Geometry: final body of the model. Coordinates: model frame, mm. Face numbers are marked on the shaded views. A direction names the side the tool comes from. Give positions to 0.01 mm unless a question says otherwise; leave off trailing zeros. Write each loop counter-clockwise with the first axis right and the second up, starting at its lowest first coordinate (ties: lowest second). Pieces come first, ordered by that corner, then holes. Notation, with made-up numbers: (12.25, -36.75) -> (42.25, -36.75) arc R27 ccw to (42.25, -12.75) -> close; hole circle Ø9 at (69, 80). An arc over 180 degrees is marked (long way). Answer in a Markdown table with one row per item. Add a question column.
Autodesk Inventor part; units mm, degrees
ref_plane "YZ Plane" through (0, 0, 0) normal (1, 0, 0) x (0, 1, 0)
ref_plane "XZ Plane" through (0, 0, 0) normal (0, 1, 0) x (-1, 0, 0)
ref_plane "XY Plane" through (0, 0, 0) normal (0, 0, 1) x (1, 0, 0)
sketch "Sketch1" plane through (0, 0, 0) normal (0, 1, 0) x (-1, 0, 0)
  circle A0 centre (0, 0) radius 9.25
  circle A1 centre (0, 0) radius 13.25
  dimension "d0" = 18.5
  dimension "d1" = 4
extrude "Extrusion1" add sketch "Sketch1" along normal blind 20
sketch "Sketch4" plane through (0, 0, 0) normal (0, -1, 0) x (1, 0, 0)
  circle A0 centre (0, 0) radius 13.25
  circle A1 centre (0, 0) radius 13.25
extrude "Extrusion2" add sketch "Sketch4" along normal blind 3
sketch "Sketch5" plane through (0, 20, 0) normal (0, 1, 0) x (1, 0, 0)
  circle A0 centre (0, 0) radius 9.25
  circle A1 centre (0, 0) radius 11.25
  dimension "d6" = 2
extrude "Extrusion3" cut sketch "Sketch5" against normal blind 3
properties part number "springPusher"
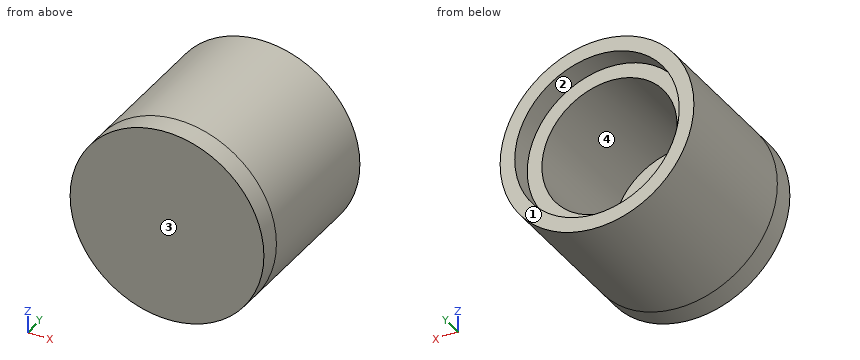
Q1. Section C-C on y = 6.5. Return loops of the section in (x, z), and give its area (3 significant figures).
Q2. Section A-A on x = -5. Return loops of the section in (y, z).
Q3. Section B-B on z = -10.5. Return loops of the section in (x, y).
Q4. Line query: probe 1 along Z at (x, y) = (0, 8); probe 2 along Z at (x, y) = (0, 18.9); probe 3 along Z at (x, y) = (-7, -0.5). Output: solid intervals per line, ascending. Write a range as from..to.
Q5. Pull-direction query (Z, two-part tool) for the marked faces 1 and 2; classes: +Z half, -Z half, draft (parallel to the pull), parting line (faces both ways), or undercut.
Q6. Contact query for flat-ended pins moving along their axis: pin 1 Ø5.5 at (x, z) = (0, -3) entering from +Y; pin 2 Ø4 at (y, z) = (8.5, 8.5) entering from -X; pin 3 Ø12 at (y, z) = (11, -6) entering from -X; pin 4 Ø4 at (y, z) = (17, 10) entering from +X. Output: stop coordinate, or through.
Q7. Access query for the marked faces 3 and 4. Directions: +Z, -Z, +X, -X, +Y, -Y. A direction counts if a zero-diameter tool reaches every point of the face in a straight line with its end or side. Return the directions, or none.
Q8. Section D-D on x = 6. Return loops of the section in (y, z), and give its area (3 significant figures).
Checks:
| question | item | result |
|---|---|---|
| 1 | outline | circle Ø26.5 at (0, 0); hole circle Ø18.5 at (0, 0) |
| 1 | area | 283 mm^2 |
| 2 | outline | (-3, -12.27) -> (20, -12.27) -> (20, -10.08) -> (17, -10.08) -> (17, -7.78) -> (0, -7.78) -> (0, 7.78) -> (17, 7.78) -> (17, 10.08) -> (20, 10.08) -> (20, 12.27) -> (-3, 12.27) -> close |
| 3 | outline | (-8.08, -3) -> (8.08, -3) -> (8.08, 20) -> (4.04, 20) -> (4.04, 17) -> (-4.04, 17) -> (-4.04, 20) -> (-8.08, 20) -> close |
| 4 | probe 1 | -13.25..-9.25, 9.25..13.25 |
| 4 | probe 2 | -13.25..-11.25, 11.25..13.25 |
| 4 | probe 3 | -11.25..11.25 |
| 5 | face 1 | draft |
| 5 | face 2 | undercut |
| 6 | pin 1 | y = 0 |
| 6 | pin 2 | x = -11.55 |
| 6 | pin 3 | x = -13.25 |
| 6 | pin 4 | x = 10.56 |
| 7 | face 3 | +Z, -Z, +X, -X, -Y |
| 7 | face 4 | +Y |
| 8 | outline | (-3, -11.81) -> (20, -11.81) -> (20, -9.52) -> (17, -9.52) -> (17, -7.04) -> (0, -7.04) -> (0, 7.04) -> (17, 7.04) -> (17, 9.52) -> (20, 9.52) -> (20, 11.81) -> (-3, 11.81) -> close |
| 8 | area | 247 mm^2 |
